Read the model definition and answer for the solid it produces. Units are mm, in the model's axes. Give positions to 0.01 mm unless a question says otherwise; leave off trailing zeros. Loops run counter-clockwise (first coordinate to the right, second up) from the corner with the lowest first, then second, coordinate; pieces in that order, holes last. Notation, with made-up numbers: (14, -21.75) -> (45, -21.75) arc R6 cw to (45, -16.75) -> close; hole circle Ø5 at (-27, 32.5). An arc over 180 degrees is marked (long way). Return JSON: item names as keys, results as strings. Group by question number.
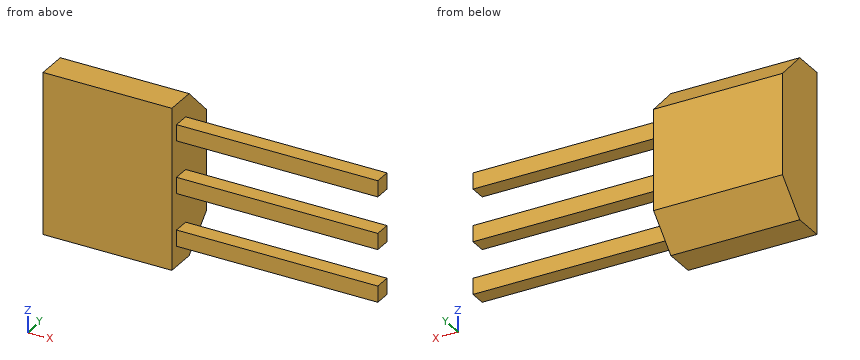
Autodesk Inventor part; units mm, degrees
ref_plane "YZ Plane" through (0, 0, 0) normal (1, 0, 0) x (0, 1, 0)
ref_plane "XZ Plane" through (0, 0, 0) normal (0, 1, 0) x (-1, 0, 0)
ref_plane "XY Plane" through (0, 0, 0) normal (0, 0, 1) x (1, 0, 0)
sketch "Skizze1" plane through (0, 0, 0) normal (1, 0, 0) x (0, 1, 0)
  line L0 (0, 0) -> (0, 4)
  line L1 (0, 4) -> (0.75, 4)
  line L2 (0.75, 4) -> (1.5, 3.25)
  line L3 (1.5, 3.25) -> (1.5, 0.75)
  line L4 (1.5, 0.75) -> (0.75, 0)
  line L5 (0.75, 0) -> (0, 0)
  point P0 (1.5, 2)
  point P1 (0, 2)
  dimension "d0" = 4
  dimension "d1" = 1.5
  dimension "d2" = 0.75
  dimension "d3" = 45
extrude "Extrusion1" add sketch "Skizze1" along normal blind 3.2
sketch "Skizze2" plane through (3.2, 0, 0) normal (1, 0, 0) x (0, 0, -1)
  line L0 (-3.1, 0.2) -> (-3.5, 0.2)
  line L1 (-3.5, 0.2) -> (-3.5, 0.6)
  line L2 (-3.5, 0.6) -> (-3.1, 0.6)
  line L3 (-3.1, 0.6) -> (-3.1, 0.2)
  line L4 (-1.8, 0.6) -> (-2.2, 0.6)
  line L5 (-2.2, 0.6) -> (-2.2, 0.2)
  line L6 (-2.2, 0.2) -> (-1.8, 0.2)
  line L7 (-1.8, 0.2) -> (-1.8, 0.6)
  line L8 (-0.9, 0.6) -> (-0.5, 0.6)
  line L9 (-0.5, 0.6) -> (-0.5, 0.2)
  line L10 (-0.5, 0.2) -> (-0.9, 0.2)
  line L11 (-0.9, 0.2) -> (-0.9, 0.6)
  line L12 (-3.5, 0.4) -> (-0.5, 0.4) construction
  line L13 (-0.75, 1.5) -> (-3.25, 1.5)
  point P0 (0, 0)
  point P1 (-2, 0.4)
  point P2 (-2, 0.6)
  point P3 (-2.2, 0.4)
  point P4 (-2, 1.5)
  dimension "d6" = 0.4
  dimension "d7" = 3
  dimension "d8" = 0.9
extrude "Extrusion2" add sketch "Skizze2" along normal blind 5
properties part number "08-04-02-008_hallSensor" material "ABS-Kunststoff(1)"
1. Straight lines are drawn through the part: line 1 (Z direction, x = 4.75, y = 0.5); line 2 (X direction, y = 0.95, z = 2.7); line 3 (Y direction, x = 5.5, z = 3.35). For each, find the intervals that lie inside material, in ascending order. Write a range as from..to.
2. Section C-C on y = 0.45 is taken. Determine the outline of the cut face in (x, z).
3. Section D-D on x = 2.5 is taken. Determine the outline of the cut face in (y, z), then the cut area to 3 significant figures.
4. Section B-B on z = 1.9 is taken. Determine the outline of the cut face in (x, y), then the cut area to 3 significant figures.
5. Section A-A on x = 5.25 is taken. Determine the outline of the cut face in (y, z), then the cut area to 3 significant figures.
Completed:
{
 "1": {"line 1": "z = 0.5..0.9, 1.8..2.2, 3.1..3.5", "line 2": "x = 0..3.2", "line 3": "y = 0.2..0.6"},
 "2": {"outline": "(0, 0) -> (3.2, 0) -> (3.2, 0.5) -> (8.2, 0.5) -> (8.2, 0.9) -> (3.2, 0.9) -> (3.2, 1.8) -> (8.2, 1.8) -> (8.2, 2.2) -> (3.2, 2.2) -> (3.2, 3.1) -> (8.2, 3.1) -> (8.2, 3.5) -> (3.2, 3.5) -> (3.2, 4) -> (0, 4) -> close"},
 "3": {"outline": "(0, 0) -> (0.75, 0) -> (1.5, 0.75) -> (1.5, 3.25) -> (0.75, 4) -> (0, 4) -> close", "area": "5.44 mm²"},
 "4": {"outline": "(0, 0) -> (3.2, 0) -> (3.2, 0.2) -> (8.2, 0.2) -> (8.2, 0.6) -> (3.2, 0.6) -> (3.2, 1.5) -> (0, 1.5) -> close", "area": "6.80 mm²"},
 "5": {"outline": "(0.2, 0.5) -> (0.6, 0.5) -> (0.6, 0.9) -> (0.2, 0.9) -> close; (0.2, 1.8) -> (0.6, 1.8) -> (0.6, 2.2) -> (0.2, 2.2) -> close; (0.2, 3.1) -> (0.6, 3.1) -> (0.6, 3.5) -> (0.2, 3.5) -> close", "area": "0.480 mm²"}
}
